from build123d import *

# Parameters (mm, degrees)
BOSS_EXTRUDE1_DEPTH                            = 24.13
CBORE_FOR_8_BUTTON_HEAD_CAP_SCREW1_D           = 4.4958
CBORE_FOR_8_BUTTON_HEAD_CAP_SCREW1_CBORE_D     = 8.73252
CBORE_FOR_8_BUTTON_HEAD_CAP_SCREW1_CBORE_DEPTH = 2.2098
CUT_EXTRUDE1_DEPTH                             = 42.512826714
CUT_EXTRUDE1_DEPTH_BACK                        = 42.512826714
SKETCH6_R                                      = 3.175
CUT_EXTRUDE2_DEPTH                             = 42.512826714
CUT_EXTRUDE2_DEPTH_BACK                        = 5.588
SKETCH7_R                                      = 8.128
FILLET1_R                                      = 0.635


with BuildPart() as part:
    # Sketch1 → Boss-Extrude1 (new body)
    with BuildSketch(Plane.XY):
        with BuildLine():
            Line((-31.75, 12.7), (31.75, 12.7))
            Line((31.75, 12.7), (31.75, -3.175))
            ThreePointArc((31.75, -3.175), (0, 1.167638116), (-31.75, -3.175))
            Line((-31.75, -3.175), (-31.75, 12.7))
        make_face()
    extrude(amount=BOSS_EXTRUDE1_DEPTH)

    # CBORE for #8 Button Head Cap Screw1 (through all)
    with Locations(Plane(origin=(0, 12.7, 0), x_dir=(1, 0, 0), z_dir=(0, 1, 0))):
        with Locations((0, -12.065)):
            CounterBoreHole(CBORE_FOR_8_BUTTON_HEAD_CAP_SCREW1_D / 2, CBORE_FOR_8_BUTTON_HEAD_CAP_SCREW1_CBORE_D / 2, CBORE_FOR_8_BUTTON_HEAD_CAP_SCREW1_CBORE_DEPTH)

    # Sketch6 → Cut-Extrude1 (cut, two sides: drawn at the far end of the back side and taken through both)
    with BuildSketch(Plane(origin=(0, 1.167638116, 0), x_dir=(-1, 0, 0), z_dir=(0, -1, 0)).offset(-CUT_EXTRUDE1_DEPTH_BACK)):
        with Locations(Location((12.7, -12.065, 0), (0, 0, 90))):
            Circle(SKETCH6_R)
        with Locations(Location((-12.7, -12.065, 0), (0, 0, 90))):
            Circle(SKETCH6_R)
    extrude(amount=CUT_EXTRUDE1_DEPTH + CUT_EXTRUDE1_DEPTH_BACK, mode=Mode.SUBTRACT)

    # Sketch7 → Cut-Extrude2 (cut, two sides: drawn at the far end of the back side and taken through both)
    with BuildSketch(Plane(origin=(0, 1.167638116, 0), x_dir=(-1, 0, 0), z_dir=(0, -1, 0)).offset(-CUT_EXTRUDE2_DEPTH_BACK)):
        with Locations(Location((12.7, -12.065, 0), (0, 0, 270))):
            Circle(SKETCH7_R)
        with Locations(Location((-12.7, -12.065, 0), (0, 0, 270))):
            Circle(SKETCH7_R)
    extrude(amount=CUT_EXTRUDE2_DEPTH + CUT_EXTRUDE2_DEPTH_BACK, mode=Mode.SUBTRACT)

    # Fillet1
    fillet1_edges = [part.edges().sort_by_distance(p)[0] for p in [
        (0, 12.7, 24.13),
        (-31.75, 4.7625, 24.13),
        (0, 1.167638116, 24.13),
        (-31.75, 4.7625, 0),
        (0, 12.7, 0),
        (31.75, 4.7625, 0),
        (0, 1.167638116, 0),
        (31.75, 4.7625, 24.13),
        (-31.75, -3.175, 12.065),
        (-31.75, 12.7, 12.065),
        (31.75, 12.7, 12.065),
        (31.75, -3.175, 12.065),
    ]]
    fillet(fillet1_edges, radius=FILLET1_R)


solid = part.part
The model under review builds one solid part; all positions refer to its coordinate system, in mm. A direction names the side the tool comes from. Round coordinates to 2 decimals unless told otherwise and drop trailing zeros. Order: outer loops, then holes, each group sorted by start corner. A loop starts at its lowest first (then second) coordinate and runs counter-clockwise, first axis right, second up. Notation, with made-up numbers: (1, 51) - (43, 51) arc R14 ccw to (43, 62) - close; hole circle Ø11 at (74.25, 28). An arc over 180 degrees is marked (long way). Use one line per item in the form item = value.
Q1. Add section A-A on x = 0. Give the boundary of the cut face in (y, z) (3 decimals).
Response values:
outline = (1.168, 0.635) arc R0.635 ccw to (1.803, 0) - (12.065, 0) arc R0.635 ccw to (12.7, 0.635) - (12.7, 7.699) - (10.49, 7.699) - (10.49, 9.817) - (1.168, 9.817) - close; (1.168, 14.313) - (10.49, 14.313) - (10.49, 16.431) - (12.7, 16.431) - (12.7, 23.495) arc R0.635 ccw to (12.065, 24.13) - (1.803, 24.13) arc R0.635 ccw to (1.168, 23.495) - close
Q2. Add section C-C on z = 2.75. Give the boundary of the cut face in (x, y) (3 decimals).
Response values:
outline = (-31.75, -2.342) arc R0.635 ccw to (-30.949, -2.955) arc R118.237 cw to (30.949, -2.955) arc R0.635 ccw to (31.75, -2.342) - (31.75, 12.065) arc R0.635 ccw to (31.115, 12.7) - (-31.115, 12.7) arc R0.635 ccw to (-31.75, 12.065) - close
Q3. To check wall thickness, follow line 1 (X direction, y = 11.25, z = 9.25); line 2 (X direction, y = 5, z = 8.5); line 3 (Z direction, x = 0, y = 11.6). State the ranges of each line that lie inside material, in increasing order.
Response values:
line_1 = -31.75 to -14.17, -11.23 to -3.34, 3.34 to 11.23, 14.17 to 31.75
line_2 = -31.75 to -20, -5.4 to 5.4, 20 to 31.75
line_3 = 0 to 7.7, 16.43 to 24.13
Q4. Add section D-D on y = 4.5. Give the boundary of the cut face in (x, z) (3 decimals), then the cut area to 3 significant figures.
Response values:
outline = (-31.75, 0.635) arc R0.635 ccw to (-31.115, 0) - (31.115, 0) arc R0.635 ccw to (31.75, 0.635) - (31.75, 23.495) arc R0.635 ccw to (31.115, 24.13) - (-31.115, 24.13) arc R0.635 ccw to (-31.75, 23.495) - close; hole circle Ø16.256 at (-12.7, 12.065); hole circle Ø4.496 at (0, 12.065); hole circle Ø16.256 at (12.7, 12.065)
area = 1,100 mm^2
Q5. Add section B-B on y = 7.75. Give the boundary of the cut face in (x, z) (3 decimals), then the cut area to 3 significant figures.
Response values:
outline = (-31.75, 0.635) arc R0.635 ccw to (-31.115, 0) - (31.115, 0) arc R0.635 ccw to (31.75, 0.635) - (31.75, 23.495) arc R0.635 ccw to (31.115, 24.13) - (-31.115, 24.13) arc R0.635 ccw to (-31.75, 23.495) - close; hole circle Ø6.35 at (-12.7, 12.065); hole circle Ø4.496 at (0, 12.065); hole circle Ø6.35 at (12.7, 12.065)
area = 1,450 mm^2
Q6. Clearance check with flat-ended pins moving along their axes: P1, Ø2.5, axis at x = -1, z = 10.5, coming from the +Y side; P2, Ø13, axis at x = -12.7, z = 12.065, coming from the +Y side; P3, Ø3.5, axis at x = 0, z = 12.065, coming from the -Y side; P4, Ø14, axis at x = 0, z = 12.065, coming from the -Y side. State where each tip first meets the part, or that it passes through.
Response values:
P1 = 10.49
P2 = 12.7
P3 = through
P4 = 1.03
Q7. Mouldability with a two-part tool opening along Z and no side actions: class faces 1 (the cylindrical face through (-15.517, 9.769, 10.6)), 2 (the flat face through (31.75, 5, 12)), 3 (the flat face through (0, 7, 24.13)) as pulls with the +Z half, pulls with the -Z half, needs draft (parallel to the pull), parting line crosses it, or undercut.
Response values:
face_1 = undercut
face_2 = needs draft
face_3 = pulls with the +Z half
Q8. Tool access review of faces 4 (the cylindrical face through (-0.568, 11.611, 7.736)), 5 (the flat face through (16.2, 6.756, 12)), 6 (the flat face through (-31.75, 5, 12)): name each direction out of +Z, -Z, +X, -X, +Y, -Y from which nothing blocks a thin tool from reaching the whole face with its end or side.
Response values:
face_4 = +Y
face_5 = -Y
face_6 = +Z, -Z, -X, +Y, -Y
